Input: part model. Units: mm. Frame: model coordinates. A direction names the side the tool comes from. Give positions to 0.01 mm unless a question says otherwise; leave off trailing zeros. Loops run counter-clockwise (first coordinate to the right, second up) from the corner with the lowest first, then second, coordinate; pieces in that order, holes last. Notation, with made-up numbers: (-36.5, 84.5) - (-29.5, 84.5) arc R7 ccw to (-29.5, 90.5) - close; hole circle Ø9 at (31, -36.75). An arc over 180 degrees is marked (long way). One line per question, with ' | ' between items. Start each with the question number.
from build123d import *

# Parameters (mm, degrees)
SKETCH1_W           = 25.4
SKETCH1_H           = 25.4
SKETCH1_W_2         = 22.225
SKETCH1_H_2         = 22.225
BOSS_EXTRUDE1_DEPTH = 863.6
SKETCH2_R           = 2.5527
CUT_EXTRUDE1_DEPTH  = 865.066785613
SKETCH3_R           = 2.5527
CUT_EXTRUDE2_DEPTH  = 865.066785613


with BuildPart() as part:
    # Sketch1 → Boss-Extrude1 (new body)
    with BuildSketch(Plane(origin=(0, 0, 0), x_dir=(1, 0, 0), z_dir=(0, 1, 0))):
        Rectangle(SKETCH1_W, SKETCH1_H)
        Rectangle(SKETCH1_W_2, SKETCH1_H_2, mode=Mode.SUBTRACT)
    extrude(amount=BOSS_EXTRUDE1_DEPTH)

    # Sketch2 → Cut-Extrude1 (cut, through all)
    with BuildSketch(Plane.XY.offset(12.7)):
        with Locations((0, 9.525)):
            Circle(SKETCH2_R)
        with Locations((0, 28.575)):
            Circle(SKETCH2_R)
    extrude(amount=-CUT_EXTRUDE1_DEPTH, mode=Mode.SUBTRACT)

    # Sketch3 → Cut-Extrude2 (cut, through all)
    with BuildSketch(Plane(origin=(12.7, 0, 0), x_dir=(0, 0, -1), z_dir=(1, 0, 0))):
        with Locations((0, 9.525)):
            Circle(SKETCH3_R)
        with Locations((0, 28.575)):
            Circle(SKETCH3_R)
        with Locations((0, 47.625)):
            Circle(SKETCH3_R)
        with Locations((0, 854.075)):
            Circle(SKETCH3_R)
        with Locations((0, 835.025)):
            Circle(SKETCH3_R)
    extrude(amount=-CUT_EXTRUDE2_DEPTH, mode=Mode.SUBTRACT)


solid = part.part
Q1. Line query: L1, parallel to Y at x = 11.8, z = 0; L2, parallel to Y at x = 0, z = 11.75; L3, parallel to X at y = 618, z = -6.25. Output: solid intervals per line, ascending. Write a range as from..to.
Q2. Draft query along Z for faces 1 (the face through (-11.112, 426, 0)), 2 (the face through (-11.3, 863.6, -0.1)), 3 (the face through (0, 426, -12.7)). Return one class per face: +Z half, -Z half, draft (parallel to the pull), parting line (faces both ways), or undercut.
Q3. Section A-A, the plane y = 549. Output: boundary loops of the cut face in (x, z).
Q4. Access query for faces 4 (the face through (11.112, 426, 0)), 5 (the face through (0, 426, 12.7)). Directions: +Z, -Z, +X, -X, +Y, -Y. A direction counts if a zero-diameter tool reaches every point of the face in a straight line with its end or side. Return the directions, or none.
Q5. First-contact query: pin 1 (3 mm diameter, centred on y = 47.625, z = 0, fed in from +X). Flat tip, straight axial feed; report the tip coordinate or a pass-through.
Solved:
1) L1: y = 0..6.97, 12.08..26.02, 31.13..45.07, 50.18..832.47, 837.58..851.52, 856.63..863.6 | L2: y = 0..6.97, 12.08..26.02, 31.13..863.6 | L3: x = -12.7..-11.11, 11.11..12.7
2) face 1: undercut | face 2: draft | face 3: -Z half
3) outline: (-12.7, -12.7) - (12.7, -12.7) - (12.7, 12.7) - (-12.7, 12.7) - close; hole (-11.11, -11.11) - (11.11, -11.11) - (11.11, 11.11) - (-11.11, 11.11) - close
4) face 4: +Y, -Y | face 5: +Z, +X, -X, +Y, -Y
5) pin 1: passes through
